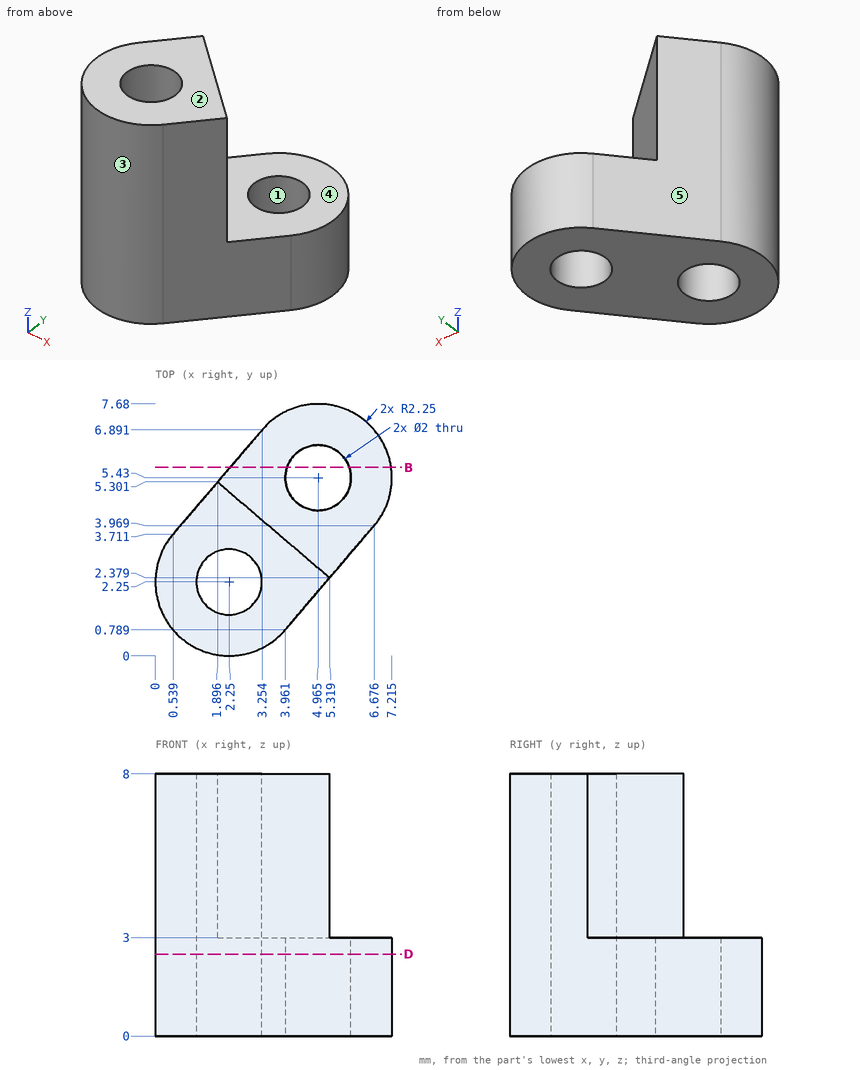
For this review, use the dimensioned drawing (mm, ordinates from the lowest corner) and the shaded views. A direction names the side the tool comes from. Coordinates: 2 decimals unless noted, no trailing zeros. Write each loop counter-clockwise with the first axis right and the second up, starting at its lowest first coordinate (ties: lowest second). Pieces come first, ordered by that corner, then holes. Notation, with made-up numbers: (-36.5, 3) - (12.5, 3) arc R19 ccw to (12.5, 24) - close; hole circle Ø2 at (23.25, 88.25). An arc over 180 degrees is marked (long way). One line per item, written item: value.
1) To check wall thickness, follow probe 1 along Y at (x, z) = (5, 1.5) (1 decimal); probe 2 along X at (y, z) = (5.43, 1.4) (1 decimal); probe 3 along Z at (x, y) = (6, 4). State the ranges of each line that lie inside material, in increasing order.
Answer sheet:
probe 1: y = 2 to 4.4, 6.4 to 7.7
probe 2: x = 2 to 4, 6 to 7.2
probe 3: z = 0 to 3
2) Insertion check: pin 1 (1.8 mm diameter, centred on x = 4.965, y = 5.43, fed in from -Z); pin 2 (3 mm diameter, centred on y = 2.5, z = 6, fed in from +X); pin 3 (2 mm diameter, centred on x = 2, z = 2, fed in from +Y) (1 decimal); pin 4 (1.5 mm diameter, centred on x = 1.5, z = 7, fed in from +Y). Each pin has a flat end and moves straight along its axis. Give the tip position at first contact, or say it passes through.
Answer sheet:
pin 1: passes through
pin 2: stops at x = 5.32
pin 3: stops at y = 6.6
pin 4: stops at y = 5.3
3) Add section B-B (y = 5.75). State the section outline as (x, z) points.
Answer sheet:
outline: (2.28, 0) - (4.02, 0) - (4.02, 3) - (2.28, 3) - close; (5.91, 0) - (7.19, 0) - (7.19, 3) - (5.91, 3) - close
4) Add section D-D (z = 2.5). Give the number of separate pieces and of enclosed holes in the cut face.
Answer sheet:
separate pieces: 1
enclosed holes: 2
5) Mouldability with a two-part tool opening along Y and no side actions: class the marked faces 1, 2 and 3 as +Y half, -Y half, draft (parallel to the pull), parting line (faces both ways), or undercut.
Answer sheet:
face 1: undercut
face 2: draft
face 3: parting line
6) For the marked faces 4 and 5, list the 3-axis set-ups (+Z, -Z, +X, -X, +Y, -Y) from which the entire face can be reached by the end or side of a thin tool; tool diameter is ignored.
Answer sheet:
face 4: +Z, +X, +Y
face 5: +Z, -Z, -X, +Y
